Geometry check sheet. Reference: the model listing, model coordinates, mm. A direction names the side the tool comes from. Coordinates: 2 decimals unless noted, no trailing zeros. Loops run counter-clockwise (first coordinate to the right, second up) from the corner with the lowest first, then second, coordinate; pieces in that order, holes last. Notation, with made-up numbers: (43, 5) - (59, 5) arc R15 cw to (59, 9) - close; hole circle Ø10 at (9, 39.5). An arc over 180 degrees is marked (long way). One line per item, written item: value.
Autodesk Inventor part; units mm, degrees
ref_plane "Work Plane2" through (2.8575, 0, 0) normal (1, 0, 0) x (0, 0, -1)
ref_plane "YZ Plane" through (0, 0, 0) normal (1, 0, 0) x (0, 1, 0)
ref_plane "XZ Plane" through (0, 0, 0) normal (0, 1, 0) x (-1, 0, 0)
ref_plane "Work Plane2" through (2.8575, 0, 0) normal (1, 0, 0) x (0, 0, -1)
sketch "Sketch6" plane through (2.8575, 0, 0) normal (1, 0, 0) x (0, 0, -1)
  line L0 (0.7654, -5.6784) -> (0.7654, -5.022)
  line L1 (-0.7638, -5.6784) -> (-0.7638, -5.0222)
  arc A0 (5.6006, 2.3498) -> (5.5837, 2.3418) centre (6.3532, 0.7382) ccw
  arc A1 (-0.7638, -5.0222) -> (0.7654, -5.022) centre (0, 0) ccw
  line L2 (0.0008, -7.62) -> (-0.2439, -7.62)
  line L3 (0.0008, -7.62) -> (0.2479, -7.62)
  arc A2 (0.2479, -7.62) -> (0.7654, -5.6784) centre (-2.309, -5.8988) ccw
  arc A3 (-0.7638, -5.6784) -> (-0.2439, -7.62) centre (2.2185, -5.9201) ccw
  arc A4 (3.5877, -3.5965) -> (3.5976, -3.5866) centre (0, 0) ccw
  line L4 (3.502, -4.5349) -> (3.1738, -3.9665)
  line L5 (2.1777, -5.2996) -> (1.8496, -4.7313)
  arc A5 (1.8496, -4.7313) -> (3.1738, -3.9665) centre (0, 0) ccw
  line L6 (3.8107, -6.5987) -> (3.5988, -6.721)
  line L7 (3.8107, -6.5987) -> (4.0247, -6.4752)
  arc A6 (4.0247, -6.4752) -> (3.502, -4.5349) centre (0.9498, -6.263) ccw
  arc A7 (2.1777, -5.2996) -> (3.5988, -6.721) centre (4.8813, -4.0177) ccw
  line L8 (5.3003, -2.1764) -> (4.7319, -1.8482)
  line L9 (4.5358, -3.5007) -> (3.9675, -3.1726)
  arc A8 (3.9675, -3.1726) -> (4.7319, -1.8482) centre (0, 0) ccw
  line L10 (6.5995, -3.8093) -> (6.4772, -4.0212)
  line L11 (6.5995, -3.8093) -> (6.7231, -3.5953)
  arc A9 (6.7231, -3.5953) -> (5.3003, -2.1764) centre (3.954, -4.949) ccw
  arc A10 (4.5358, -3.5007) -> (6.4772, -4.0212) centre (6.2362, -1.0388) ccw
  line L12 (5.6784, 0.7654) -> (5.022, 0.7654)
  line L13 (5.6784, -0.7638) -> (5.0222, -0.7638)
  arc A11 (5.0222, -0.7638) -> (5.022, 0.7654) centre (0, 0) ccw
  line L14 (7.62, 0.0008) -> (7.62, -0.2439)
  line L15 (7.62, 0.0008) -> (7.62, 0.2479)
  arc A12 (7.62, 0.2479) -> (5.6784, 0.7654) centre (5.8988, -2.309) ccw
  arc A13 (5.6784, -0.7638) -> (7.62, -0.2439) centre (5.9201, 2.2185) ccw
  line L16 (4.5349, 3.502) -> (3.9665, 3.1738)
  line L17 (5.2996, 2.1777) -> (4.7313, 1.8496)
  arc A14 (4.7313, 1.8496) -> (3.9665, 3.1738) centre (0, 0) ccw
  line L18 (6.5987, 3.8107) -> (6.721, 3.5988)
  line L19 (6.5987, 3.8107) -> (6.4752, 4.0247)
  arc A15 (6.4752, 4.0247) -> (4.5349, 3.502) centre (6.263, 0.9498) ccw
  arc A16 (5.2996, 2.1777) -> (6.721, 3.5988) centre (4.0177, 4.8813) ccw
  line L20 (2.1764, 5.3003) -> (1.8482, 4.7319)
  line L21 (3.5007, 4.5358) -> (3.1726, 3.9675)
  arc A17 (3.1726, 3.9675) -> (1.8482, 4.7319) centre (0, 0) ccw
  line L22 (3.8093, 6.5995) -> (4.0212, 6.4772)
  line L23 (3.8093, 6.5995) -> (3.5953, 6.7231)
  arc A18 (3.5953, 6.7231) -> (2.1764, 5.3003) centre (4.949, 3.954) ccw
  arc A19 (3.5007, 4.5358) -> (4.0212, 6.4772) centre (1.0388, 6.2362) ccw
  line L24 (-0.7654, 5.6784) -> (-0.7654, 5.022)
  line L25 (0.7638, 5.6784) -> (0.7638, 5.0222)
  arc A20 (0.7638, 5.0222) -> (-0.7654, 5.022) centre (0, 0) ccw
  line L26 (-0.0008, 7.62) -> (0.2439, 7.62)
  line L27 (-0.0008, 7.62) -> (-0.2479, 7.62)
  arc A21 (-0.2479, 7.62) -> (-0.7654, 5.6784) centre (2.309, 5.8988) ccw
  arc A22 (0.7638, 5.6784) -> (0.2439, 7.62) centre (-2.2185, 5.9201) ccw
  line L28 (-3.502, 4.5349) -> (-3.1738, 3.9665)
  line L29 (-2.1777, 5.2996) -> (-1.8496, 4.7313)
  arc A23 (-1.8496, 4.7313) -> (-3.1738, 3.9665) centre (0, 0) ccw
  line L30 (-3.8107, 6.5987) -> (-3.5988, 6.721)
  line L31 (-3.8107, 6.5987) -> (-4.0247, 6.4752)
  arc A24 (-4.0247, 6.4752) -> (-3.502, 4.5349) centre (-0.9498, 6.263) ccw
  arc A25 (-2.1777, 5.2996) -> (-3.5988, 6.721) centre (-4.8813, 4.0177) ccw
  line L32 (-5.3003, 2.1764) -> (-4.7319, 1.8482)
  line L33 (-4.5358, 3.5007) -> (-3.9675, 3.1726)
  arc A26 (-3.9675, 3.1726) -> (-4.7319, 1.8482) centre (0, 0) ccw
  line L34 (-6.5995, 3.8093) -> (-6.4772, 4.0212)
  line L35 (-6.5995, 3.8093) -> (-6.7231, 3.5953)
  arc A27 (-6.7231, 3.5953) -> (-5.3003, 2.1764) centre (-3.954, 4.949) ccw
  arc A28 (-4.5358, 3.5007) -> (-6.4772, 4.0212) centre (-6.2362, 1.0388) ccw
  line L36 (-5.6784, -0.7654) -> (-5.022, -0.7654)
  line L37 (-5.6784, 0.7638) -> (-5.0222, 0.7638)
  arc A29 (-5.0222, 0.7638) -> (-5.022, -0.7654) centre (0, 0) ccw
  line L38 (-7.62, -0.0008) -> (-7.62, 0.2439)
  line L39 (-7.62, -0.0008) -> (-7.62, -0.2479)
  arc A30 (-7.62, -0.2479) -> (-5.6784, -0.7654) centre (-5.8988, 2.309) ccw
  arc A31 (-5.6784, 0.7638) -> (-7.62, 0.2439) centre (-5.9201, -2.2185) ccw
  line L40 (-4.5349, -3.502) -> (-3.9665, -3.1738)
  line L41 (-5.2996, -2.1777) -> (-4.7313, -1.8496)
  arc A32 (-4.7313, -1.8496) -> (-3.9665, -3.1738) centre (0, 0) ccw
  line L42 (-6.5987, -3.8107) -> (-6.721, -3.5988)
  line L43 (-6.5987, -3.8107) -> (-6.4752, -4.0247)
  arc A33 (-6.4752, -4.0247) -> (-4.5349, -3.502) centre (-6.263, -0.9498) ccw
  arc A34 (-5.2996, -2.1777) -> (-6.721, -3.5988) centre (-4.0177, -4.8813) ccw
  line L44 (-2.1764, -5.3003) -> (-1.8482, -4.7319)
  line L45 (-3.5007, -4.5358) -> (-3.1726, -3.9675)
  arc A35 (-3.1726, -3.9675) -> (-1.8482, -4.7319) centre (0, 0) ccw
  line L46 (-3.8093, -6.5995) -> (-4.0212, -6.4772)
  line L47 (-3.8093, -6.5995) -> (-3.5953, -6.7231)
  arc A36 (-3.5953, -6.7231) -> (-2.1764, -5.3003) centre (-4.949, -3.954) ccw
  arc A37 (-3.5007, -4.5358) -> (-4.0212, -6.4772) centre (-1.0388, -6.2362) ccw
  arc A38 (-1.8482, -4.7319) -> (-0.7638, -5.0222) centre (0, 0) ccw
  line L48 (-2.0137, 5.0155) -> (-0.7654, 5.3502)
  line L49 (0.7638, 5.3503) -> (2.0123, 5.0161)
  line L50 (3.3367, 4.2516) -> (4.2507, 3.3379)
  line L51 (5.0155, 2.0137) -> (5.3502, 0.7654)
  line L52 (5.3503, -0.7638) -> (5.0161, -2.0123)
  line L53 (4.2516, -3.3367) -> (3.3379, -4.2507)
  line L54 (2.0137, -5.0155) -> (0.7654, -5.3502)
  line L55 (-0.7638, -5.3503) -> (-2.0123, -5.0161)
  line L56 (-3.3367, -4.2516) -> (-4.2507, -3.3379)
  line L57 (-5.0155, -2.0137) -> (-5.3502, -0.7654)
  line L58 (-5.3503, 0.7638) -> (-5.0161, 2.0123)
  line L59 (-4.2516, 3.3367) -> (-3.3379, 4.2507)
  circle A39 centre (0, 0) radius 5.0531
  point P0 (0, 0)
  point P1 (-4.2516, 3.3367)
  dimension "d94" = 360
extrude "Extrusion19" add sketch "Sketch6" against normal blind 11.4554 contours A2 L3 L2 A3 L1 A1 L0 | L0 A1 A38 A35 L45 L56 L40 A32 L41 L57 L36 A29 L37 L58 L32 A26 L33 L59 L28 A23 L29 L48 L24 A20 L25 L49 L20 A17 L21 L50 L16 A14 L17 L51 L12 A11 L13 L52 L8 A8 L9 L53 L4 A5 L5 L54 | L5 A5 L4 A6 L7 L6 A7 | L1 L55 L44 A38 | L44 A36 L47 L46 A37 L45 A35 | L9 A8 L8 A9 L11 L10 A10 | L40 A33 L43 L42 A34 L41 A32 | L13 A11 L12 A12 L15 L14 A13 | L36 A30 L39 L38 A31 L37 A29 | L17 A14 L16 A15 L19 L18 A16 | L32 A27 L35 L34 A28 L33 A26 | L21 A17 L20 A18 L23 L22 A19 | L28 A24 L31 L30 A25 L29 A23 | L25 A20 L24 A21 L27 L26 A22 | A39
sketch "Sketch7" plane through (-8.5979, 0, 0) normal (-1, 0, 0) x (0, 0, 1)
  circle A0 centre (0, 0) radius 1.625
  dimension "d104" = 3.25
extrude "Extrusion20" cut sketch "Sketch7" against normal blind 2540
sketch "Sketch8" plane through (-8.5979, 0, 0) normal (-1, 0, 0) x (0, 0, 1)
  circle A0 centre (0, 0) radius 5.08
  line L0 (-3.3367, 4.2516) -> (-4.2507, 3.3379)
  arc A1 (-4.2507, 3.3379) -> (-3.3367, 4.2516) centre (-4.209, 4.2103) ccw
  line L1 (-3.3367, 4.2516) -> (-3.5007, 4.5358)
  line L2 (-4.2507, 3.3379) -> (-3.3367, 4.2516)
  arc A2 (-5.3502, 0.7654) -> (-5.0155, 2.0137) centre (-5.7503, 1.5417) ccw
  line L3 (-5.3502, 0.7654) -> (-5.0155, 2.0137)
  arc A3 (-5.0161, -2.0123) -> (-5.3503, -0.7638) centre (-5.7507, -1.54) ccw
  line L4 (-5.0161, -2.0123) -> (-5.3503, -0.7638)
  arc A4 (-3.3379, -4.2507) -> (-4.2516, -3.3367) centre (-4.2103, -4.209) ccw
  line L5 (-3.3379, -4.2507) -> (-4.2516, -3.3367)
  arc A5 (-0.7654, -5.3502) -> (-2.0137, -5.0155) centre (-1.5417, -5.7503) ccw
  line L6 (-0.7654, -5.3502) -> (-2.0137, -5.0155)
  arc A6 (2.0123, -5.0161) -> (0.7638, -5.3503) centre (1.54, -5.7507) ccw
  line L7 (2.0123, -5.0161) -> (0.7638, -5.3503)
  arc A7 (4.2507, -3.3379) -> (3.3367, -4.2516) centre (4.209, -4.2103) ccw
  line L8 (4.2507, -3.3379) -> (3.3367, -4.2516)
  arc A8 (5.3502, -0.7654) -> (5.0155, -2.0137) centre (5.7503, -1.5417) ccw
  line L9 (5.3502, -0.7654) -> (5.0155, -2.0137)
  arc A9 (5.0161, 2.0123) -> (5.3503, 0.7638) centre (5.7507, 1.54) ccw
  line L10 (5.0161, 2.0123) -> (5.3503, 0.7638)
  arc A10 (3.3379, 4.2507) -> (4.2516, 3.3367) centre (4.2103, 4.209) ccw
  line L11 (3.3379, 4.2507) -> (4.2516, 3.3367)
  arc A11 (0.7654, 5.3502) -> (2.0137, 5.0155) centre (1.5417, 5.7503) ccw
  line L12 (0.7654, 5.3502) -> (2.0137, 5.0155)
  arc A12 (-2.0123, 5.0161) -> (-0.7638, 5.3503) centre (-1.54, 5.7507) ccw
  line L13 (-2.0123, 5.0161) -> (-0.7638, 5.3503)
  dimension "d107" = 10.16
  dimension "d110" = 360
extrude "Extrusion21" cut sketch "Sketch8" against normal blind 2540 contours A8 L9 | A7 L8 | A6 L7 | A5 L6 | A4 L5 | A3 L4 | A2 L3 | A1 L0 | A12 L13 | A11 L12 | A10 L11 | A9 L10
properties part number "Alligator_Pinion (2)"
(1) Cross-section at A-A on y = 0. Record the cut outline in (x, z) (1 decimal), and give its area (3 significant figures).
Reply:
outline: (-8.6, -7.6) - (2.9, -7.6) - (2.9, -1.6) - (-8.6, -1.6) - close; (-8.6, 1.6) - (2.9, 1.6) - (2.9, 7.6) - (-8.6, 7.6) - close
area: 137 mm2
(2) Access from +Z, -Z, +X, -X, +Y, -Y to the whole of each face (thin tool, end or side, straight path). Record for faces 5 (the face through (-2.79, -5.48, -3.93)), 6 (the face through (-2.79, -6.141, 2.777)), 7 (the face through (-2.79, -2.755, 6.123)), 8 (the face through (-2.79, 6.123, 2.755)).
Reply:
face 5: -Z, +X, -X
face 6: +X, -X, -Y
face 7: +Z, +X, -X
face 8: +X, -X, +Y
(3) Cross-section at C-C on z = -2.5. Record the cut outline in (x, y).
Reply:
outline: (-8.6, -5.83) - (2.86, -5.83) - (2.86, 5.83) - (-8.6, 5.83) - close
(4) Go/stop test with flat-tipped pins: pin 1 Ø6 at (x, y) = (-3.5, -5) entering from -Z; pin 2 Ø3 at (y, z) = (0, 0) entering from +X; pin 3 Ø1.5 at (x, y) = (-5.5, -4.5) entering from +Z. Record where each tip stops, or that it passes through.
Reply:
pin 1: z = -6.72
pin 2: through
pin 3: z = 6.63
(5) Material ranges on probe 1 along Y at (x, z) = (-4.5, 0) (3 decimals); probe 2 along Y at (x, z) = (-3.75, 5); probe 3 along Y at (x, z) = (-5.25, -3.5), recorded low to high. Write a range as from..to.
Reply:
probe 1: -7.62..-1.625, 1.625..7.62
probe 2: -3.76..-1.99, -1.09..1.09, 1.99..3.76
probe 3: -6.67..-4.53, -3.7..3.7, 4.53..6.67
(6) Release check for a two-part mould opening along Z. For faces 1 (the face through (-2.79, 2.755, -6.123)), 2 (the face through (-2.95, -0.99, -1.29)), 3 (the face through (-2.79, -6.123, -2.755)), 4 (the face through (2.858, 2, 0)) record: pulls with the +Z half, pulls with the -Z half, needs draft (parallel to the pull), parting line crosses it, or undercut.
Reply:
face 1: pulls with the -Z half
face 2: undercut
face 3: undercut
face 4: needs draft
